from build123d import *

# Parameters (mm, degrees)
F0_W     = 15.8
F0_H     = 14
F1_DEPTH = 13.4
F2_R     = 6.4
F3_DEPTH = 4
F4_R     = 5.920321
F4_R_2   = 5.413043
F5_DEPTH = 7
F6_R     = 0.7
F7_DEPTH = 10


with BuildPart() as f1:
    # F0 (on Front) → F1 (new body)
    with BuildSketch(Plane.XZ):
        with Locations((7.9, 7)):
            Rectangle(F0_W, F0_H)
    extrude(amount=F1_DEPTH)

    # F2 (on face) → F3 (join)
    with BuildSketch(Plane.XZ.offset(13.4)):
        with Locations((7.9, 7)):
            Circle(F2_R)
    extrude(amount=F3_DEPTH)

    # F4 (on face) → F5 (cut)
    with BuildSketch(Plane.XZ.offset(17.4)):
        with Locations((7.9, 7)):
            Circle(F4_R)
        with Locations((7.9, 7)):
            Circle(F4_R_2, mode=Mode.SUBTRACT)
    extrude(amount=-F5_DEPTH, mode=Mode.SUBTRACT)

    # F6 (on face) → F7 (cut)
    with BuildSketch(Plane.XZ.offset(17.4)):
        with Locations((5.964432, 9.765608)):
            Circle(F6_R)
        with Locations((9.884015, 9.676018)):
            Circle(F6_R)
        with Locations((6.255601, 7.100292)):
            Circle(F6_R)
        with Locations((9.436062, 7.055497)):
            Circle(F6_R)
    extrude(amount=-F7_DEPTH, mode=Mode.SUBTRACT)


solid = f1.part
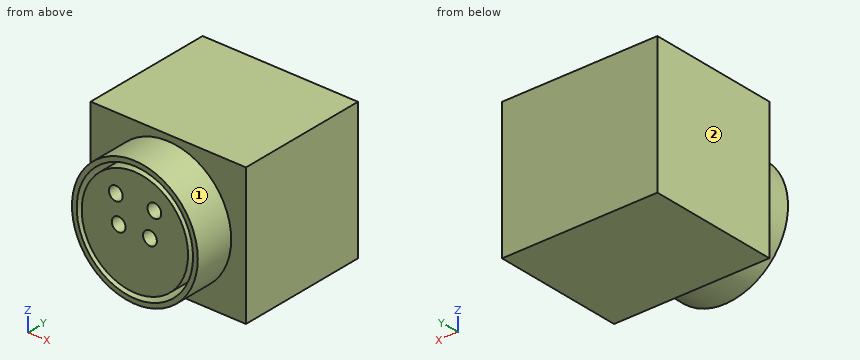
Geometry: final body of the model. Coordinates: model frame, mm. Face numbers are marked on the shaded views. A direction names the side the tool comes from. Round coordinates to 2 decimals unless told otherwise and drop trailing zeros. Order: outer loops, then holes, each group sorted by start corner. A loop starts at its lowest first (then second) coordinate and runs counter-clockwise, first axis right, second up. Notation, with made-up numbers: (-8.5, 38.25) -> (30.5, 38.25) arc R23 ccw to (30.5, 74.25) -> close; hole circle Ø6 at (23.25, -33.75). An arc over 180 degrees is marked (long way). Put each result on its own line as item: value. Start each with the question number.
Q1. Section C-C on z = 3. Return the cut outline in (x, y), and give its area (3 significant figures).
Q2. Section B-B on y = -14.75. Return the cut outline in (x, z).
Q3. Reachability of the marked faces 1 and 2 from +Z, -Z, +X, -X, +Y, -Y: full face, straight path, thin tool, end or side. Return the list, or none.
Q4. Line query: probe 1 along X at (y, z) = (-14.5, 10); probe 2 along X at (y, z) = (-13.25, 4); probe 3 along Z at (x, y) = (9, -16). Output: solid intervals per line, ascending.
Q5. Section A-A on x = 7.9. Return the cut outline in (y, z).
Q6. First-contact query: pin 1 (0.8 mm diameter, centred on x = 9.88, z = 9.68, fed in from -Y); pin 2 (2 mm diameter, centred on y = -15.5, z = 2.5, fed in from +X). Flat tips, straight axial feed; report the tip coordinate or a pass-through.
Ans:
1. outline: (0, -13.4) -> (2.9, -13.4) -> (2.9, -17.4) -> (3.54, -17.4) -> (3.54, -10.4) -> (4.25, -10.4) -> (4.25, -17.4) -> (11.55, -17.4) -> (11.55, -10.4) -> (12.26, -10.4) -> (12.26, -17.4) -> (12.9, -17.4) -> (12.9, -13.4) -> (15.8, -13.4) -> (15.8, 0) -> (0, 0) -> close
1. area: 242 mm2
2. outline: circle Ø12.8 at (7.9, 7); circle Ø10.83 at (7.9, 7); hole circle Ø11.84 at (7.9, 7); hole circle Ø1.4 at (5.96, 9.77); hole circle Ø1.4 at (6.26, 7.1); hole circle Ø1.4 at (9.44, 7.06); hole circle Ø1.4 at (9.88, 9.68)
3. face 1: -Y
3. face 2: +Z, -Z, -X, +Y, -Y
4. probe 1: x = 2.25 to 2.8, 3.39 to 5.3, 6.62 to 9.26, 10.5 to 12.41, 13 to 13.55
4. probe 2: x = 0 to 2.8, 3.39 to 12.41, 13 to 15.8
4. probe 3: z = 0.7 to 1.18, 1.7 to 6.51, 7.6 to 12.3, 12.82 to 13.3
5. outline: (-17.4, 0.6) -> (-13.4, 0.6) -> (-13.4, 0) -> (0, 0) -> (0, 14) -> (-13.4, 14) -> (-13.4, 13.4) -> (-17.4, 13.4) -> (-17.4, 12.92) -> (-10.4, 12.92) -> (-10.4, 12.41) -> (-17.4, 12.41) -> (-17.4, 1.59) -> (-10.4, 1.59) -> (-10.4, 1.08) -> (-17.4, 1.08) -> close
6. pin 1: stops at y = -7.4
6. pin 2: stops at x = 13.26
